from build123d import *

# Parameters (mm, degrees)
BOSS_EXTRUDE1_DEPTH     = 4
SKETCH2_R               = 2.7
CUT_EXTRUDE2_DEPTH      = 8.662003654
CUT_EXTRUDE2_DEPTH_BACK = 8.662003654


with BuildPart() as part:
    # Sketch1 → Boss-Extrude1 (new, symmetric)
    with BuildSketch(Plane(origin=(0, 0, 0), x_dir=(1, 0, 0), z_dir=(0, 1, 0))):
        Polygon((4.278165495, -2.47), (4.278165495, 2.47), (0, 4.94), (-4.278165495, 2.47), (-4.278165495, -2.47), (0, -4.94), align=None)
    extrude(amount=BOSS_EXTRUDE1_DEPTH, both=True)

    # SurfaceCut1
    split(bisect_by=Plane.XY.offset(-0.5), keep=Keep.TOP)

    # Sketch2 → Cut-Extrude2 (cut, two sides)
    with BuildSketch(Plane.XY) as cut_extrude2_sk:
        with Locations(Location((0, 0, 0), (0, 0, 270))):
            Circle(SKETCH2_R)
    extrude(amount=CUT_EXTRUDE2_DEPTH, mode=Mode.SUBTRACT)
    extrude(cut_extrude2_sk.sketch, amount=-CUT_EXTRUDE2_DEPTH_BACK, mode=Mode.SUBTRACT)


solid = part.part
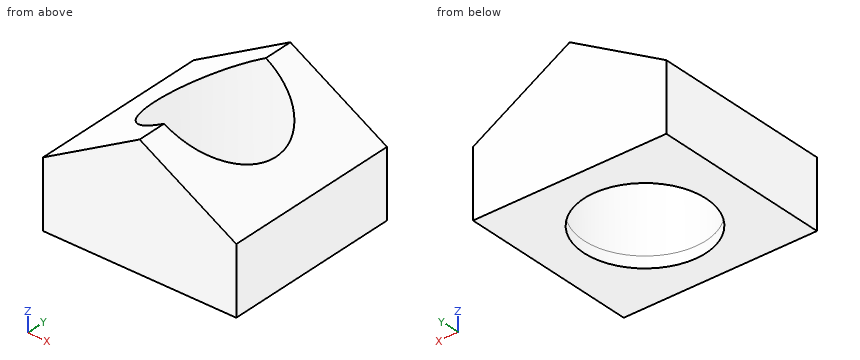
Here's how the part is built. I have some questions about the finished solid (model axes, mm). Give positions to 0.01 mm unless a question says otherwise; leave off trailing zeros. Loops run counter-clockwise (first coordinate to the right, second up) from the corner with the lowest first, then second, coordinate; pieces in that order, holes last. Notation, with made-up numbers: (-15.5, -37.75) -> (-6.5, -37.75) arc R38 ccw to (-6.5, 1.25) -> close; hole circle Ø10 at (19, 46.5). An arc over 180 degrees is marked (long way). One line per item, written item: value.
Q1. I'm going to push flat-ended pins straight in: pin 1 Ø3 at (y, z) = (-1.5, 3) entering from +X; pin 2 Ø4.5 at (x, y) = (0, 0) entering from +Z. Where does each tip first touch, or does it pass through?
Answers follow:
pin 1: x = 4.28
pin 2: through
Q2. If I drill on line 1 along X through (y, z) = (0, 1.4); line 2 along Y through (x, z) = (-0.25, 0); line 3 along Y through (x, z) = (-1, 4.05), over which ranges is the centre line in solid material (lowest first)?
Answers follow:
line 1: -4.28 to -2.7, 2.7 to 4.28
line 2: -4 to -2.69, 2.69 to 4
line 3: -4 to -2.51, 2.51 to 4
Q3. Suppose I cut it at B-B on z = 3.8. Please give me the cut outline in (x, y).
Answers follow:
outline: (-1.97, -4) -> (1.97, -4) -> (1.97, -1.84) arc R2.7 cw to (-1.97, -1.84) -> close; (-1.97, 1.84) arc R2.7 cw to (1.97, 1.84) -> (1.97, 4) -> (-1.97, 4) -> close
Q4. Suppose I cut it at A-A on y = -1.25. Please give me the cut outline in (x, z).
Answers follow:
outline: (-4.28, -0.5) -> (-2.39, -0.5) -> (-2.39, 3.56) -> (-4.28, 2.47) -> close; (2.39, -0.5) -> (4.28, -0.5) -> (4.28, 2.47) -> (2.39, 3.56) -> close
Q5. Suppose I cut it at D-D on x = -3.25. Please give me the cut outline in (y, z), then the cut area to 3 significant figures.
Answers follow:
outline: (-4, -0.5) -> (4, -0.5) -> (4, 3.06) -> (-4, 3.06) -> close
area: 28.5 mm^2
Q6. Suppose I cut it at C-C on z = 0.55. Please give me the cut outline in (x, y), then the cut area to 3 significant figures.
Answers follow:
outline: (-4.28, -4) -> (4.28, -4) -> (4.28, 4) -> (-4.28, 4) -> close; hole circle Ø5.4 at (0, 0)
area: 45.5 mm^2
